The drawing under review shows one solid part. Ordinate dimensions are in mm from its lowest x, y, z. A direction names the side the tool comes from. Round coordinates to 2 decimals unless told otherwise and drop trailing zeros. Write each loop counter-clockwise with the first axis right and the second up, starting at its lowest first coordinate (ties: lowest second). Pieces come first, ordered by that corner, then holes.
Item 1: To check wall thickness, follow L1, parallel to Y at x = 2.15, z = 7.5 (1 decimal); L2, parallel to Z at x = 7, y = 7; L3, parallel to Z at x = 23.5, y = 9.5. State the ranges of each line that lie inside material, in increasing order.
Item 2: Machinability: for the marked faces 1, 2 and 3, which of the approach directions +Z, -Z, +X, -X, +Y, -Y give a long, thin tool a straight path to every point of the face, cutting with its end or side? Answer none if there is none.
Item 3: Add section A-A (x = 6). Give the boundary of the cut face in (y, z).
Item 4: Clearance check with flat-ended pins moving along their axes: pin 1 Ø6.5 at (y, z) = (5.48, 7.5) entering from -X; pin 2 Ø5.5 at (y, z) = (5.5, 9) entering from +X. State where each tip first meets the part, or that it passes through.
Item 5: Draft analysis for pull direction Y (two halves, no side actions). For the marked faces 4, 5 and 6, state which applies: +Y half, -Y half, draft (parallel to the pull), parting line (faces both ways), or undercut.
Item 6: Add section C-C (z = 2.75). Give the boundary of the cut face in (x, y).
Item 7: Add section D-D (x = 22). Give the boundary of the cut face in (y, z), plus the area to 3 significant figures.
Item 8: Add section B-B (y = 6.25). Give the boundary of the cut face in (x, z) (1 decimal).
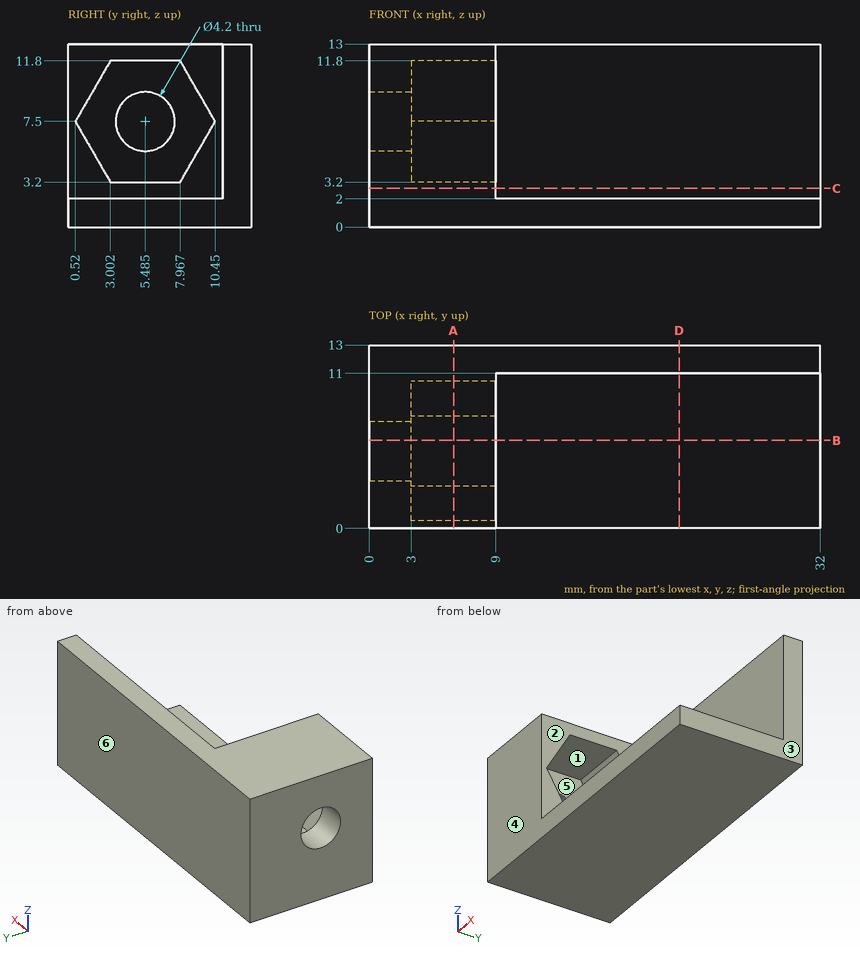
Numbers:
1. L1: y = 0 to 3.4, 7.6 to 13
1. L2: z = 0 to 3.2, 11.8 to 13
1. L3: z = 0 to 2
2. face 1: +X
2. face 2: +Z, +X, -Y
2. face 3: +Z, -Z, +X, +Y, -Y
3. outline: (0, 0) - (13, 0) - (13, 13) - (0, 13) - close; hole (0.52, 7.5) - (3, 3.2) - (7.97, 3.2) - (10.45, 7.5) - (7.97, 11.8) - (3, 11.8) - close
4. pin 1: stops at x = 0
4. pin 2: stops at x = 3
5. face 4: -Y half
5. face 5: undercut
5. face 6: +Y half
6. outline: (0, 0) - (9, 0) - (9, 11) - (32, 11) - (32, 13) - (0, 13) - close
7. outline: (0, 0) - (13, 0) - (13, 13) - (11, 13) - (11, 2) - (0, 2) - close
7. area: 48.0 mm2
8. outline: (0, 0) - (32, 0) - (32, 2) - (9, 2) - (9, 3.2) - (3, 3.2) - (3, 5.5) - (0, 5.5) - close; (0, 9.5) - (3, 9.5) - (3, 11.8) - (9, 11.8) - (9, 13) - (0, 13) - close
